Could you check a few things on this model? Use its own coordinates, in mm. A direction names the side the tool comes from. Coordinates: 2 decimals unless noted, no trailing zeros. Loops run counter-clockwise (first coordinate to the right, second up) from the corner with the lowest first, then second, coordinate; pieces in that order, holes last. Notation, with made-up numbers: (62.5, 67) - (91.5, 67) arc R30 cw to (91.5, 98) - close; hole circle Ø8 at (58.5, 17). An arc over 180 degrees is marked (long way). Put each result on its own line as item: value. Start each with the question number.
```python
from build123d import *

# Parameters (mm, degrees)
SKETCH1_R  = 1
BODY_DEPTH = 1
FILLET1_R  = 0.2
FILLET2_R  = 0.5


with BuildPart() as part:
    # Sketch1 → Body (new body)
    with BuildSketch(Plane.XY):
        with BuildLine():
            Line((-1.25, -9.280254038), (-1.25, -13.258334542))
            ThreePointArc((-1.25, -13.258334542), (-4.197569907, -12.606259086), (-6.907964473, -11.276923892))
            Line((-6.907964473, -11.276923892), (-7.592035527, -7.397364163))
            ThreePointArc((-7.592035527, -7.397364163), (0, 10.6), (7.592035527, -7.397364163))
            Line((7.592035527, -7.397364163), (6.907964473, -11.276923892))
            ThreePointArc((6.907964473, -11.276923892), (4.197569907, -12.606259086), (1.25, -13.258334542))
            Line((1.25, -13.258334542), (1.25, -9.280254038))
            ThreePointArc((1.25, -9.280254038), (0, 8.13), (-1.25, -9.280254038))
        make_face()
        with Locations(Location((4.25, -10.439750506, 0), (0, 0, 180))):
            Circle(SKETCH1_R, mode=Mode.SUBTRACT)
        with Locations((-4.25, -10.439750506)):
            Circle(SKETCH1_R, mode=Mode.SUBTRACT)
    extrude(amount=-BODY_DEPTH)

    # Fillet1
    fillet1_edges = [part.edges().sort_by_distance(p)[0] for p in [
        (-6.907964473, -11.276923892, -0.5),
        (6.907964473, -11.276923892, -0.5),
    ]]
    fillet(fillet1_edges, radius=FILLET1_R)

    # Fillet2
    fillet2_edges = [part.edges().sort_by_distance(p)[0] for p in [
        (-7.592035527, -7.397364163, -0.5),
        (7.592035527, -7.397364163, -0.5),
    ]]
    fillet(fillet2_edges, radius=FILLET2_R)


solid = part.part
```
(1) I want a section at C-C on z = -0.45. List the corners of the cut face in (x, y) for me.
(2) I want a section at D-D on x = -7.25. List the corners of the cut face in (y, z) for me, and give its area (3 significant figures).
(3) For pin 1 Ø1.8 at (x, y) = (-4.25, -10.44) entering from +Z; pin 2 Ø0.5 at (y, z) = (-12, -0.5) entering from -X; pin 3 Ø0.5 at (y, z) = (-10.5, -0.5) entering from +X, each with a flat end and sliding along its axis, tell me the tip position at first contact or that it passes through.
(4) I want a section at A-A on x = 4.25. List the corners of the cut face in (y, z) for me.
(5) Which directions (+Z, -Z, +X, -X, +Y, -Y) give clear straight access to the entire face, cutting with the end or side of a thin tool? Please do faces 1 (the cylindrical face through (-4.116, -12.634, -0.493)), 2 (the flat face through (1.25, -11.3, -0.5)).
(6) I need wall thicknesses on L1, parallel to X at y = -11.25, z = -0.35; L2, parallel to Y at x = -4.25, z = -0.7; L3, parallel to X at y = -10.75, z = -0.75. Which ranges of each line are inside material? Lowest first, please. Write a range as [from, to].
(7) If we mould it in two halves opening along Y, with no side actions, what happens to faces 3 (the cylindrical face through (-4.38, -9.45, -0.49)), 4 (the flat face through (-1.25, -11.2, -0.5)), 5 (the cylindrical face through (4.195, -12.607, -0.493))? For each: pulls with the +Y half, pulls with the -Y half, needs draft (parallel to the pull), parting line crosses it, or undercut.
(8) I want a section at B-B on y = -4.25. List the corners of the cut face in (x, z) for me.
Answer sheet:
1. outline: (-7.7, -7.29) arc R0.5 cw to (-7.57, -7.55) - (-6.92, -11.19) arc R0.2 ccw to (-6.83, -11.32) arc R12.7 ccw to (-1.25, -13.26) - (-1.25, -9.28) arc R8.75 cw (long way) to (1.25, -9.28) - (1.25, -13.26) arc R12.7 ccw to (6.83, -11.32) arc R0.2 ccw to (6.92, -11.19) - (7.57, -7.55) arc R0.5 cw to (7.7, -7.29) arc R10.6 ccw (long way) to start; hole circle Ø2 at (-4.25, -10.44); hole circle Ø2 at (4.25, -10.44)
2. outline: (-9.34, -1) - (-5.52, -1) - (-5.52, 0) - (-9.34, 0) - close; (4.28, -1) - (7.73, -1) - (7.73, 0) - (4.28, 0) - close
2. area: 7.27 mm^2
3. pin 1: passes through
3. pin 2: stops at x = -6.12
3. pin 3: stops at x = 7.09
4. outline: (-12.59, -1) - (-11.44, -1) - (-11.44, 0) - (-12.59, 0) - close; (-9.44, -1) - (-8.27, -1) - (-8.27, 0) - (-9.44, 0) - close; (7.03, -1) - (9.71, -1) - (9.71, 0) - (7.03, 0) - close
5. face 1: +Z, -Z, -X, -Y
5. face 2: +Z, -Z, -Y
6. L1: x = [-6.9, -4.84], [-3.66, -1.25], [1.25, 3.66], [4.84, 6.9]
6. L2: y = [-12.59, -11.44], [-9.44, -8.27], [7.03, 9.71]
6. L3: x = [-7, -5.2], [-3.3, -1.25], [1.25, 3.3], [5.2, 7]
7. face 3: undercut
7. face 4: needs draft
7. face 5: pulls with the -Y half
8. outline: (-9.71, -1) - (-7.96, -1) - (-7.96, 0) - (-9.71, 0) - close; (7.96, -1) - (9.71, -1) - (9.71, 0) - (7.96, 0) - close
